Part model, mm, in its own coordinate system. A direction names the side the tool comes from. Coordinates: 2 decimals unless noted, no trailing zeros. Loops run counter-clockwise (first coordinate to the right, second up) from the corner with the lowest first, then second, coordinate; pieces in that order, holes last. Notation, with made-up numbers: (-35, -12.5) - (-18, -12.5) arc R3 ccw to (-18, -8.5) - close; hole circle Ø1 at (51.5, 44). An arc over 180 degrees is marked (long way). Use a Markdown table: item, result. Add a question column.
1. Band-saw the part on A-A, the plane z = -17. Give the cut face in (x, y), plus the area to 3 significant figures.
2. Band-saw the part on B-B, the plane x = 107. Give the cut face in (y, z).
3. Wall check: probe 1 along X at (y, z) = (8.5, -2.5); probe 2 along Z at (x, y) = (109, 1.5); probe 3 along Y at (x, z) = (53, 78). Give the ranges that are in metal, low to high. Write a range as [from, to].
4. 3-axis set-ups, long thin cutter, end or side, ignore diameter. For faces 1 (the flat face through (-2, 2.5, 80)), 2 (the flat face through (117, 2.5, 1)), 3 (the flat face through (112.5, 5, 80)), 4 (the flat face through (2, 7.5, 80)), 5 (the flat face through (117, 7.5, -1)): which of +Z, -Z, +X, -X, +Y, -Y reach the whole face in a straight line?
5. Drop flat-ended pins along their axis: pin 1 (11 mm diameter, centred on x = 118.5, z = -23.5, fed in from -Y); pin 2 (8 mm diameter, centred on x = 12.5, z = 80, fed in from +Y); pin 3 (1.5 mm diameter, centred on y = 5.5, z = 82, fed in from +X). Give the stop position or say it passes through.
Autodesk Inventor part; units mm, degrees
ref_plane "YZ Plane" through (0, 0, 0) normal (1, 0, 0) x (0, 1, 0)
ref_plane "XZ Plane" through (0, 0, 0) normal (0, 1, 0) x (-1, 0, 0)
ref_plane "XY Plane" through (0, 0, 0) normal (0, 0, 1) x (1, 0, 0)
sketch "Sketch1" plane through (0, 0, 0) normal (0, 1, 0) x (-1, 0, 0)
  line L0 (-112.5, 75) -> (112.5, 75)
  line L1 (112.5, 75) -> (112.5, -75)
  line L2 (112.5, -75) -> (-112.5, -75)
  line L3 (-112.5, -75) -> (-112.5, 75)
  line L4 (-112.5, 75) -> (112.5, -75) construction
  line L5 (112.5, 75) -> (-112.5, -75) construction
  point P0 (0, 0)
  dimension "d0" = 225
  dimension "d1" = 150
extrude "Extrusion1" add sketch "Sketch1" along normal blind 10
sketch "Sketch2" plane through (112.5, 0, 75) normal (1, 0, 0) x (0, 0, -1)
  line L0 (0, 2.5) -> (150, 2.5)
  line L1 (150, 2.5) -> (150, 7.5)
  line L2 (150, 7.5) -> (0, 7.5)
  line L3 (0, 7.5) -> (0, 2.5)
  point P0 (75, 0)
  point P1 (0, 5)
  dimension "d4" = 150
  dimension "d5" = 5
extrude "Extrusion2" add sketch "Sketch2" along normal blind 10
sketch "Sketch3" plane through (-112.5, 0, 75) normal (0, 0, 1) x (1, 0, 0)
  line L0 (0, 2.5) -> (225, 2.5)
  line L1 (225, 2.5) -> (225, 7.5)
  line L2 (225, 7.5) -> (0, 7.5)
  line L3 (0, 7.5) -> (0, 2.5)
  point P0 (112.5, 0)
  dimension "d8" = 225
  dimension "d9" = 5
extrude "Extrusion3" add sketch "Sketch3" along normal blind 10
properties part number "TSU_Baseplate"
Geometry check:
| question | item | result |
|---|---|---|
| 1 | outline | (-112.5, 0) - (112.5, 0) - (112.5, 2.5) - (122.5, 2.5) - (122.5, 7.5) - (112.5, 7.5) - (112.5, 10) - (-112.5, 10) - close |
| 1 | area | 2,300 mm^2 |
| 2 | outline | (0, -75) - (10, -75) - (10, 75) - (7.5, 75) - (7.5, 85) - (2.5, 85) - (2.5, 75) - (0, 75) - close |
| 3 | probe 1 | x = [-112.5, 112.5] |
| 3 | probe 2 | z = [-75, 75] |
| 3 | probe 3 | y = [2.5, 7.5] |
| 4 | face 1 | +Z, +X, -X, -Y |
| 4 | face 2 | +Z, -Z, +X, -Y |
| 4 | face 3 | +Z, +X, +Y, -Y |
| 4 | face 4 | +Z, +X, -X, +Y |
| 4 | face 5 | +Z, -Z, +X, +Y |
| 5 | pin 1 | stops at y = 2.5 |
| 5 | pin 2 | stops at y = 7.5 |
| 5 | pin 3 | stops at x = 112.5 |
